Design review of the part built by this model. Coordinates are the model's own, in mm. A direction names the side the tool comes from. Give positions to 0.01 mm unless a question says otherwise; leave off trailing zeros. Write each loop counter-clockwise with the first axis right and the second up, starting at its lowest first coordinate (ties: lowest second). Pieces come first, ordered by that corner, then holes. Notation, with made-up numbers: M 81,58 L 94,58 A28 cw 94,94 Z; hole C -13,-11.5 d9. An arc over 180 degrees is marked long. Use a Markdown table: item, result. Add a question column.
```python
from build123d import *

# Parameters (mm, degrees)
SKETCH1_W            = 40
SKETCH1_H            = 30
BOSS_EXTRUDE1_DEPTH  = 1
SKETCH2_W            = 8
SKETCH2_H            = 3
BOSS_EXTRUDE2_DEPTH  = 8
M3_CLEARANCE_HOLE1_D = 3.4
BOSS_EXTRUDE3_DEPTH  = 5
SKETCH8_W            = 2
SKETCH8_H            = 10
BOSS_EXTRUDE4_DEPTH  = 10
FILLET1_R            = 1


with BuildPart() as part:
    # Sketch1 → Boss-Extrude1 (new, symmetric)
    with BuildSketch(Plane(origin=(0, 0, 0), x_dir=(1, 0, 0), z_dir=(0, 1, 0))):
        with Locations((20, 15)):
            Rectangle(SKETCH1_W, SKETCH1_H)
    extrude(amount=BOSS_EXTRUDE1_DEPTH, both=True)

    # Sketch2 → Boss-Extrude2 (add)
    with BuildSketch(Plane(origin=(0, 1, 0), x_dir=(1, 0, 0), z_dir=(0, 1, 0))):
        with Locations((4, 1.5)):
            Rectangle(SKETCH2_W, SKETCH2_H)
        with Locations((36, 1.5)):
            Rectangle(SKETCH2_W, SKETCH2_H)
    extrude(amount=BOSS_EXTRUDE2_DEPTH)

    # M3 Clearance Hole1 (through all)
    with Locations(Plane(origin=(0, 0, -3), x_dir=(-1, 0, 0), z_dir=(0, 0, -1))):
        with Locations((-4, 5), (-36, 5)):
            Hole(M3_CLEARANCE_HOLE1_D / 2)

    # Sketch7 → Boss-Extrude3 (add)
    with BuildSketch(Plane.XY):
        Polygon((1.5, -1), (1.5, -11), (38.5, -11), (38.5, -1), (36.5, -1), (36.5, -9), (3.5, -9), (3.5, -1), align=None)
    extrude(amount=-BOSS_EXTRUDE3_DEPTH)

    # Sketch8 → Boss-Extrude4 (add)
    with BuildSketch(Plane(origin=(0, 0, -5), x_dir=(-1, 0, 0), z_dir=(0, 0, -1))):
        with Locations((-37.5, -6)):
            Rectangle(SKETCH8_W, SKETCH8_H)
        with Locations((-2.5, -6)):
            Rectangle(SKETCH8_W, SKETCH8_H)
    extrude(amount=BOSS_EXTRUDE4_DEPTH)

    # Fillet1
    fillet1_edges = [part.edges().sort_by_distance(p)[0] for p in [
        (3.5, -11, -10),
        (2.5, -11, -15),
        (1.5, -6, -15),
        (2.5, -1, -15),
        (0.75, -1, 0),
        (39.25, -1, 0),
        (38.5, -1, -7.5),
        (38.5, -11, -7.5),
        (1.5, -11, -7.5),
        (1.5, -1, -7.5),
        (1.5, -6, 0),
        (38.5, -6, 0),
        (40, 0, -30),
        (0, 0, -30),
        (36.5, -11, -10),
        (38.5, -6, -15),
        (37.5, -11, -15),
        (37.5, -1, -15),
        (20, -11, -5),
    ]]
    fillet(fillet1_edges, radius=FILLET1_R - 0.0001)  # a hair under: the kernel refuses the full size


solid = part.part
```
(1) Wall thickness on L1, parallel to Y at x = 36, z = -1.75; L2, parallel to Y at x = 20.5, z = -3.5; L3, parallel to X at y = -2, z = -3.25: over which ranges is each line inside the solid? List them lowest first.
(2) Add section D-D on x = 13. Give the boundary of the cut face in (y, z).
(3) Add section C-C on y = -6. Give the boundary of the cut face in (x, z), then the cut area to 3 significant figures.
(4) Add section B-B on y = 5. Give the boundary of the cut face in (x, z), then the cut area to 3 significant figures.
(5) Add section A-A on x = 4. Give the boundary of the cut face in (y, z).
(6) Machinability: for faces 5 (the cylindrical face through (20.245, -10.715, -4.699)), 6 (the cylindrical face through (38.215, -6.437, -0.301)), 7 (the flat face through (38.5, -6, -7)), 8 (the cylindrical face through (38.215, -5.944, -14.699)), which of the approach directions +Z, -Z, +X, -X, +Y, -Y give a long, thin tool a straight path to every point of the face, cutting with its end or side? Answer none if there is none.
(7) For pin 1 (6.5 mm diameter, centred on y = -5, z = -5.5, fed in from -X); pin 2 (0.8 mm diameter, centred on x = 37, y = -8, fed in from -Z); pin 3 (6 mm diameter, centred on x = 11.5, z = -19.5, fed in from -Y), all flat-tipped, find the tip position at first contact; note any pin that passes through.
(8) The part is to be moulded in two halves that separate along Y. For faces 1 (the flat face through (20, 0, 0)), 2 (the cylindrical face through (2.9, -10.6, -14.8)), 3 (the flat face through (3.5, -6, -8)), 4 (the flat face through (20, -9, -2)), say which applies: released by +Y, released by -Y, zero draft, split by the parting line, or undercut.
From the geometry:
| question | item | result |
|---|---|---|
| 1 | L1 | y = -11 to -9, -1 to 3.3, 6.7 to 9 |
| 1 | L2 | y = -11 to -9, -1 to 1 |
| 1 | L3 | x = 1.5 to 3.5, 36.5 to 38.5 |
| 2 | outline | M -11,-4 A1 ccw -10,-5 L -9,-5 L -9,0 L -11,0 Z; M -1,-30 L 1,-30 L 1,0 L -1,0 Z |
| 3 | outline | M 1.5,-14 A1 ccw 2.5,-15 L 3.5,-15 L 3.5,0 L 2.5,0 A1 ccw 1.5,-1 Z; M 36.5,-15 L 37.5,-15 A1 ccw 38.5,-14 L 38.5,-1 A1 ccw 37.5,0 L 36.5,0 Z |
| 3 | area | 59.1 mm^2 |
| 4 | outline | M 0,-3 L 2.3,-3 L 2.3,0 L 0,0 Z; M 5.7,-3 L 8,-3 L 8,0 L 5.7,0 Z; M 32,-3 L 34.3,-3 L 34.3,0 L 32,0 Z; M 37.7,-3 L 40,-3 L 40,0 L 37.7,0 Z |
| 4 | area | 27.6 mm^2 |
| 5 | outline | M -11,-4 A1 ccw -10,-5 L -9,-5 L -9,0 L -11,0 Z; M -1,-30 L 1,-30 L 1,-3 L 3.3,-3 L 3.3,0 L -1,0 Z; M 6.7,-3 L 9,-3 L 9,0 L 6.7,0 Z |
| 6 | face 5 | -Z, -Y |
| 6 | face 6 | +Z, +X, -Y |
| 6 | face 7 | +Z, -Z, +X, -Y |
| 6 | face 8 | -Z, +X, -Y |
| 7 | pin 1 | stops at x = 1.47 |
| 7 | pin 2 | stops at z = -15 |
| 7 | pin 3 | stops at y = -1 |
| 8 | face 1 | zero draft |
| 8 | face 2 | released by -Y |
| 8 | face 3 | undercut |
| 8 | face 4 | undercut |
